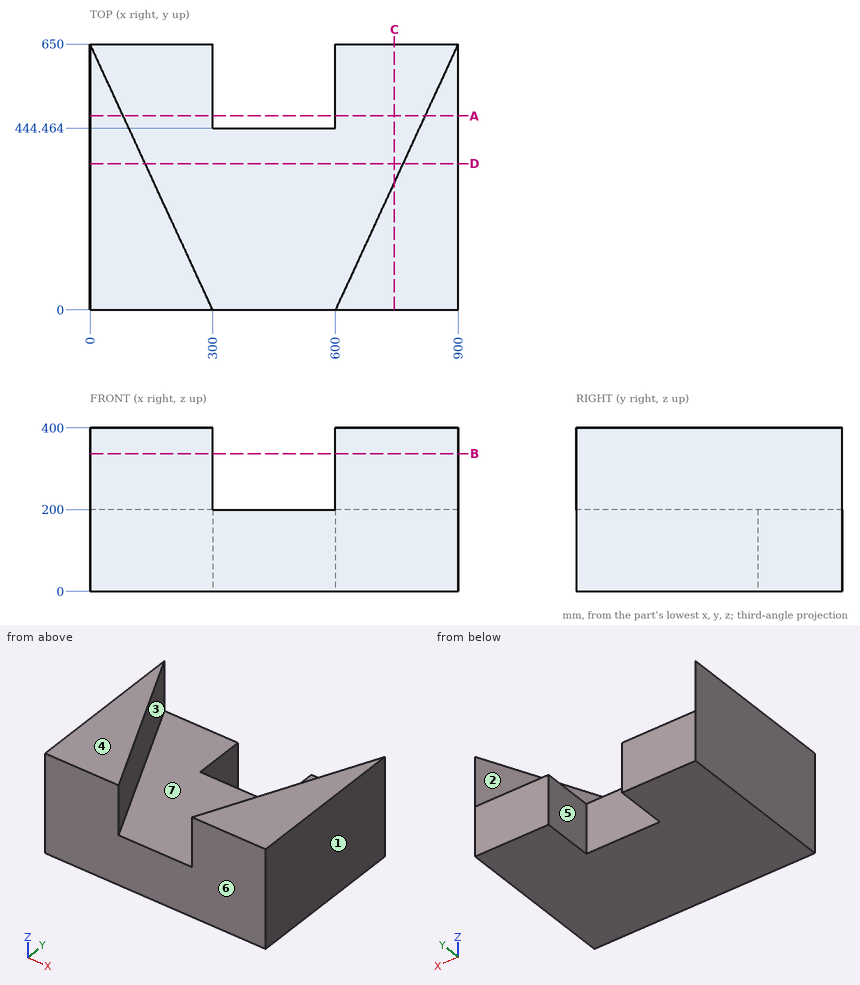
Geometry check sheet. Reference: drawing and pictorial views, mm from the part's lowest x, y, z. A direction names the side the tool comes from. Coordinates: 2 decimals unless noted, no trailing zeros. Order: outer loops, then holes, each group sorted by start corner. A loop starts at its lowest first (then second) coordinate and runs counter-clockwise, first axis right, second up. Notation, with made-up numbers: M -22.5,38 L 11.5,38 A15 ccw 11.5,59 Z; hole C 44,53.25 d3. An arc over 180 degrees is marked long. Return JSON: item names as keys, results as strings.
1) Cross-section at A-A, the plane y = 474.5. Record the boundary of the cut face in (x, z), and give its area (3 significant figures).
Answer list:
{"outline": "M 0,0 L 300,0 L 300,200 L 81,200 L 81,400 L 0,400 Z; M 600,0 L 900,0 L 900,400 L 819,400 L 819,200 L 600,200 Z", "area": "152,000 mm2"}
2) Cross-section at B-B, the plane z = 337. Record the boundary of the cut face in (x, y), and give its area (3 significant figures).
Answer list:
{"outline": "M 0,0 L 300,0 L 0,650 Z; M 600,0 L 900,0 L 900,650 Z", "area": "195,000 mm2"}
3) Release check for a two-part mould opening along X. For the marked faces 1, 2, 3 and 4 record: +X half, -X half, draft (parallel to the pull), parting line (faces both ways), or undercut.
Answer list:
{"face 1": "+X half", "face 2": "undercut", "face 3": "undercut", "face 4": "draft"}
4) Cross-section at D-D, the plane y = 357.5. Record the boundary of the cut face in (x, z), and give its area (3 significant figures).
Answer list:
{"outline": "M 0,0 L 900,0 L 900,400 L 765,400 L 765,200 L 135,200 L 135,400 L 0,400 Z", "area": "234,000 mm2"}
5) Gauge pin test, flat end, axial feed: pin 1 (1.5 mm diameter, centred on x = 94.5, y = 496, fed in from +Z). Record the tip position at first contact, or that the pin passes through.
Answer list:
{"pin 1": "z = 200"}
6) Cross-section at C-C, the plane x = 744. Record the boundary of the cut face in (y, z), and give its area (3 significant figures).
Answer list:
{"outline": "M 0,0 L 650,0 L 650,200 L 312,200 L 312,400 L 0,400 Z", "area": "192,000 mm2"}
7) Thickness scan on L1, parallel to X at y = 549.5, z = 186.5; L2, parallel to Z at x = 459, y = 70; L3, parallel to Y at x = 326.5, z = 149.5 (1 decimal). Record the ranges inside material, lowest first. Write a range as [from, to].
Answer list:
{"L1": "[0, 300], [600, 900]", "L2": "[0, 200]", "L3": "[0, 444.5]"}
8) Access from +Z, -Z, +X, -X, +Y, -Y to the whole of each face (thin tool, end or side, straight path). Record for the marked faces 5, 6 and 7.
Answer list:
{"face 5": "+Z, -Z, +Y", "face 6": "+Z, -Z, +X, -X, -Y", "face 7": "+Z, +Y"}
